Geometry: final body of the model. Coordinates: model frame, mm. A direction names the side the tool comes from. Coordinates: 2 decimals unless noted, no trailing zeros. Write each loop counter-clockwise with the first axis right and the second up, starting at its lowest first coordinate (ties: lowest second). Pieces come first, ordered by that corner, then holes. Notation, with made-up numbers: M -7,22.5 L 14,22.5 A20 cw 14,39.5 Z; hole C 68,-35 d5. An arc over 180 degrees is marked long. Write item = value, one per line. Start each with the question number.
Item 1: First-contact query: pin 1 Ø4 at (y, z) = (-42.5, 3.5) entering from +X; pin 2 Ø2 at (x, z) = (59.5, 5.5) entering from +Y; pin 3 Ø1 at (x, y) = (49.5, -62.5) entering from +Z. Flat tips, straight axial feed; report the tip coordinate or a pass-through.
Item 2: Section A-A on z = 8. Output: boundary loops of the cut face in (x, y), plus the area to 3 significant figures.
Item 3: Section D-D on x = 55. Output: boundary loops of the cut face in (y, z).
Item 4: Section C-C on z = 13.5. Output: boundary loops of the cut face in (x, y).
Item 5: Section B-B on y = -59. Output: boundary loops of the cut face in (x, z), plus the area to 4 significant figures.
Item 6: Reachability of faces 1 (the flat face through (58, -76, 10)), 2 (the flat face through (47.25, -45, 3)), 3 (the flat face through (53.75, -64, 7)) from +Z, -Z, +X, -X, +Y, -Y: full face, straight path, thin tool, end or side. Return the list, or none.
Item 7: Pull-direction query (Y, two-part tool) for faces 4 (the flat face through (45.5, -76, 10)), 5 (the flat face through (54.4, -64.1, 5)); classes: +Y half, -Y half, draft (parallel to the pull), parting line (faces both ways), or undercut.
Item 8: Ray query, L1, parallel to Y at x = 51, z = 6.5; L2, parallel to X at y = -63.5, z = 8.75; L3, parallel to X at y = -79.5, z = 10.25. Return the intervals inside material, ascending. Write a range as [from, to].
from build123d import *

# Parameters (mm, degrees)
SKETCH_W        = 22.5
SKETCH_H        = 66
PAD_DEPTH       = 15
SKETCH001_W     = 12.5
SKETCH001_H     = 75
SKETCH001_W_2   = 4.6
SKETCH001_H_2   = 4.6
POCKET_DEPTH    = 10
SKETCH002_W     = 7
SKETCH002_H     = 7
POCKET001_DEPTH = 5.8
SKETCH004_W     = 1.1
SKETCH004_H     = 4
POCKET002_DEPTH = 10
SKETCH005_W     = 4
SKETCH005_H     = 1.3
POCKET003_DEPTH = 10
SKETCH007_W     = 19.75
SKETCH007_H     = 26.5
SKETCH007_W_2   = 17.25
POCKET004_DEPTH = 20


with BuildPart() as part:
    # Sketch → Pad (new body)
    with BuildSketch(Plane.XY):
        with Locations((51.75, -67)):
            Rectangle(SKETCH_W, SKETCH_H)
    extrude(amount=PAD_DEPTH)

    # Sketch001 (on DatumPlane) → Pocket (cut)
    with BuildSketch(Plane.XY.offset(15)):
        with Locations((51.75, -57.5)):
            Rectangle(SKETCH001_W, SKETCH001_H)
        with Locations((51.75, -64)):
            Rectangle(SKETCH001_W_2, SKETCH001_H_2, mode=Mode.SUBTRACT)
    extrude(amount=-POCKET_DEPTH, mode=Mode.SUBTRACT)

    # Sketch002 (on DatumPlane) → Pocket001 (cut)
    with BuildSketch(Plane.XY.offset(15)):
        with Locations((51.5, -63.5)):
            Rectangle(SKETCH002_W, SKETCH002_H)
    extrude(amount=-POCKET001_DEPTH, mode=Mode.SUBTRACT)

    # Sketch004 (on DatumPlane) → Pocket002 (cut)
    with BuildSketch(Plane.XY.offset(15)):
        with Locations((51.75, -64)):
            Rectangle(SKETCH004_W, SKETCH004_H)
    extrude(amount=-POCKET002_DEPTH, mode=Mode.SUBTRACT)

    # Sketch005 (on DatumPlane) → Pocket003 (cut)
    with BuildSketch(Plane.XY.offset(15)):
        with Locations((51.75, -64)):
            Rectangle(SKETCH005_W, SKETCH005_H)
    extrude(amount=-POCKET003_DEPTH, mode=Mode.SUBTRACT)

    # Sketch007 (on DatumPlane) → Pocket004 (cut)
    with BuildSketch(Plane.XY.offset(15)):
        with Locations((66.125, -42.25)):
            Rectangle(SKETCH007_W, SKETCH007_H)
        with Locations((38.625, -42.25)):
            Rectangle(SKETCH007_W_2, SKETCH007_H)
    extrude(amount=-POCKET004_DEPTH, mode=Mode.SUBTRACT)


solid = part.part
Responses:
q1.pin_1 = 56.25
q1.pin_2 = -55.5
q1.pin_3 = 9.2
q2.outline = M 40.5,-100 L 63,-100 L 63,-55.5 L 58,-55.5 L 58,-95 L 45.5,-95 L 45.5,-55.5 L 40.5,-55.5 Z; M 49.45,-66.3 L 54.05,-66.3 L 54.05,-61.7 L 49.45,-61.7 Z; hole M 49.75,-64.65 L 51.2,-64.65 L 51.2,-66 L 52.3,-66 L 52.3,-64.65 L 53.75,-64.65 L 53.75,-63.35 L 52.3,-63.35 L 52.3,-62 L 51.2,-62 L 51.2,-63.35 L 49.75,-63.35 Z
q2.area = 520 mm²
q3.outline = M -100,0 L -34,0 L -34,5 L -95,5 L -95,15 L -100,15 Z
q4.outline = M 40.5,-100 L 63,-100 L 63,-55.5 L 58,-55.5 L 58,-95 L 45.5,-95 L 45.5,-55.5 L 40.5,-55.5 Z
q5.outline = M 40.5,0 L 63,0 L 63,15 L 58,15 L 58,5 L 45.5,5 L 45.5,15 L 40.5,15 Z
q5.area = 212.5 mm²
q6.face_1 = +Z, +Y
q6.face_2 = +Z, -Z, -X, +Y
q6.face_3 = +Z
q7.face_4 = draft
q7.face_5 = undercut
q8.L1 = [-100, -95], [-66.3, -64.65], [-63.35, -61.7]
q8.L2 = [40.5, 45.5], [49.45, 49.75], [53.75, 54.05], [58, 63]
q8.L3 = [40.5, 45.5], [58, 63]
